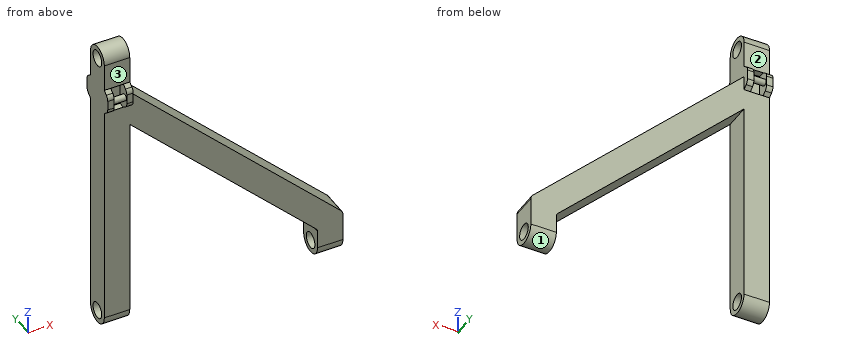
from build123d import *

# Parameters (mm, degrees)
CROQUIS1_R                 = 12.5
SALIENTE_EXTRUIR1_DEPTH    = 40
SALIENTE_EXTRUIR2_DEPTH    = 40
CORTAR_EXTRUIR2_DEPTH      = 45
CORTAR_EXTRUIR2_DEPTH_BACK = 45
CROQUIS4_R                 = 12.5
CROQUIS6_W                 = 20
CROQUIS6_H                 = 40
CORTAR_EXTRUIR3_DEPTH      = 20
CROQUIS7_R                 = 5
SALIENTE_EXTRUIR3_DEPTH    = 20


with BuildPart() as part:
    # Croquis1 → Saliente-Extruir1 (new body)
    with BuildSketch(Plane(origin=(0, 0, 0), x_dir=(0, 0, -1), z_dir=(1, 0, 0))):
        with BuildLine():
            ThreePointArc((0, 20), (-20, 0), (0, -20))
            Line((0, -20), (42.5, -20))
            Line((42.5, -20), (47, -26))
            ThreePointArc((47, -26), (50.527864045, -28.94427191), (55, -30))
            Line((55, -30), (70, -30))
            ThreePointArc((70, -30), (74.472135955, -28.94427191), (78, -26))
            Line((78, -26), (82.5, -20))
            Line((82.5, -20), (438, -20))
            ThreePointArc((438, -20), (458, 0), (438, 20))
            Line((438, 20), (82.5, 20))
            Line((82.5, 20), (78, 26))
            ThreePointArc((78, 26), (74.472135955, 28.94427191), (70, 30))
            Line((70, 30), (55, 30))
            ThreePointArc((55, 30), (50.527864045, 28.94427191), (47, 26))
            Line((47, 26), (42.5, 20))
            Line((42.5, 20), (0, 20))
        make_face()
        Circle(CROQUIS1_R, mode=Mode.SUBTRACT)
        with Locations(Location((438, 0, 0), (0, 0, 180))):
            Circle(CROQUIS1_R, mode=Mode.SUBTRACT)
    extrude(amount=SALIENTE_EXTRUIR1_DEPTH)

    # Croquis2 → Saliente-Extruir2 (add)
    with BuildSketch(Plane(origin=(0, 20, 0), x_dir=(1, 0, 0), z_dir=(0, 1, 0))):
        with BuildLine():
            Line((40, 116.134954918), (40, 60))
            Line((40, 60), (372.016025575, 386.906530798))
            ThreePointArc((372.016025575, 386.906530798), (374.223888978, 390.169590656), (375, 394.032215687))
            Line((375, 394.032215687), (375, 458))
            Line((375, 458), (335, 458))
            Line((335, 458), (335, 438.09469359))
            Line((335, 438.09469359), (335, 409.297101222))
            ThreePointArc((335, 409.297101222), (334.49922902, 406.80481537), (333.074646857, 404.699387623))
            Line((333.074646857, 404.699387623), (40, 116.134954918))
        make_face()
    extrude(amount=-SALIENTE_EXTRUIR2_DEPTH)

    # Croquis4 → Cortar-Extruir2 (cut, two sides: drawn at the far end of the back side and taken through both)
    with BuildSketch(Plane(origin=(375, 0, 0), x_dir=(0, 0, -1), z_dir=(1, 0, 0)).offset(-CORTAR_EXTRUIR2_DEPTH_BACK)):
        with Locations(Location((438, 0, 0), (0, 0, 180))):
            Circle(CROQUIS4_R)
        with BuildLine():
            Line((438, 20), (458, 20))
            Line((458, 20), (498.77405459, 20))
            Line((498.77405459, 20), (498.77405459, -20))
            Line((498.77405459, -20), (438, -20))
            ThreePointArc((438, -20), (458, 0), (438, 20))
        make_face()
    extrude(amount=CORTAR_EXTRUIR2_DEPTH + CORTAR_EXTRUIR2_DEPTH_BACK, mode=Mode.SUBTRACT)

    # Croquis6 → Cortar-Extruir3 (cut)
    with BuildSketch(Plane(origin=(0, 30, 0), x_dir=(1, 0, 0), z_dir=(0, 1, 0))):
        with Locations((20, 62.5)):
            Rectangle(CROQUIS6_W, CROQUIS6_H)
    cortar_extruir3 = extrude(amount=-CORTAR_EXTRUIR3_DEPTH, mode=Mode.SUBTRACT)

    # Croquis7 → Saliente-Extruir3 (add)
    with BuildSketch(Plane(origin=(10, 0, 0), x_dir=(0, 0, -1), z_dir=(1, 0, 0))):
        with Locations(Location((62.5, 24, 0), (0, 0, 180))):
            Circle(CROQUIS7_R)
    saliente_extruir3 = extrude(amount=SALIENTE_EXTRUIR3_DEPTH)

    # Simetr_a1: Cortar-Extruir3, Saliente-Extruir3 across plane
    add(cortar_extruir3.mirror(Plane.ZX), mode=Mode.SUBTRACT)
    add(saliente_extruir3.mirror(Plane.ZX))


solid = part.part
The listing builds one solid part. Answer for the finished solid, in the listing's coordinates (mm). Face numbers are marked on the shaded views. A direction names the side the tool comes from. Coordinates: 2 decimals unless noted, no trailing zeros. Order: outer loops, then holes, each group sorted by start corner. A loop starts at its lowest first (then second) coordinate and runs counter-clockwise, first axis right, second up.
Q1. Given P1, Ø1, axis at y = 6.5, z = -393, coming from the +X side; P2, Ø12, axis at y = -15.5, z = -310.5, coming from the +X side; P3, Ø20, axis at x = 16.5, z = -20, coming from the +Y side, each flat-ended and moving along its own axis, determine where each tip first touches the part or whether it passes through.
Q2. A cutting plane is placed at C-C, the plane x = 93. Write down the section's boundary in (y, z), and give its area (3 significant figures).
Q3. Which of the six approach directions +Z, -Z, +X, -X, +Y, -Y give full straight-line access (tool end or side, diameter ignored) to the marked faces 1, 2 and 3?
Q4. A cutting plane is placed at A-A, the plane y = 0. Write down the section's boundary in (x, z).
Q5. A cutting plane is placed at B-B, the plane z = -298.5. Write down the section's boundary in (x, y), and give its area (3 significant figures).
Q6. Consider line 1 (Z direction, x = 20.5, y = 8); line 2 (Y direction, x = 356.5, z = -438); line 3 (Z direction, x = 38.5, y = -4.5). Determine where each line is inside the solid, lowest interval first.
Answers follow:
1. P1: stops at x = 374.99
1. P2: stops at x = 300.51
1. P3: stops at y = 20
2. outline: (-20, -168.32) - (20, -168.32) - (20, -112.18) - (-20, -112.18) - close
2. area: 2,250 mm2
3. face 1: -Z, +X, -X
3. face 2: +Z, +X, -X, +Y
3. face 3: +Z, +X, -X, -Y
4. outline: (0, -458) - (40, -458) - (40, -450.5) - (0, -450.5) - close; (0, -425.5) - (40, -425.5) - (40, -116.13) - (333.07, -404.7) arc R6.45 cw to (335, -409.3) - (335, -425.5) - (375, -425.5) - (375, -394.03) arc R10 ccw to (372.02, -386.91) - (40, -60) - (40, -12.5) - (0, -12.5) - close; (0, 12.5) - (40, 12.5) - (40, 20) - (0, 20) - close; (335, -458) - (375, -458) - (375, -450.5) - (335, -450.5) - close
5. outline: (0, -20) - (40, -20) - (40, 20) - (0, 20) - close; (225.22, -20) - (282.23, -20) - (282.23, 20) - (225.22, 20) - close
5. area: 3,880 mm2
6. line 1: z = -456.33 to -447.6, -428.4 to -9.6, 9.6 to 18.33
6. line 2: y = -20 to -12.5, 12.5 to 20
6. line 3: z = -457.49 to -449.66, -426.34 to -11.66, 11.66 to 19.49
